Could you check a few things on this drawing? It's one solid part, dimensions in mm from its lowest x, y, z. A direction names the side the tool comes from. Give positions to 0.01 mm unless a question says otherwise; leave off trailing zeros. Order: outer loops, then holes, each group sorted by start corner. A loop starts at its lowest first (then second) coordinate and runs counter-clockwise, first axis right, second up.
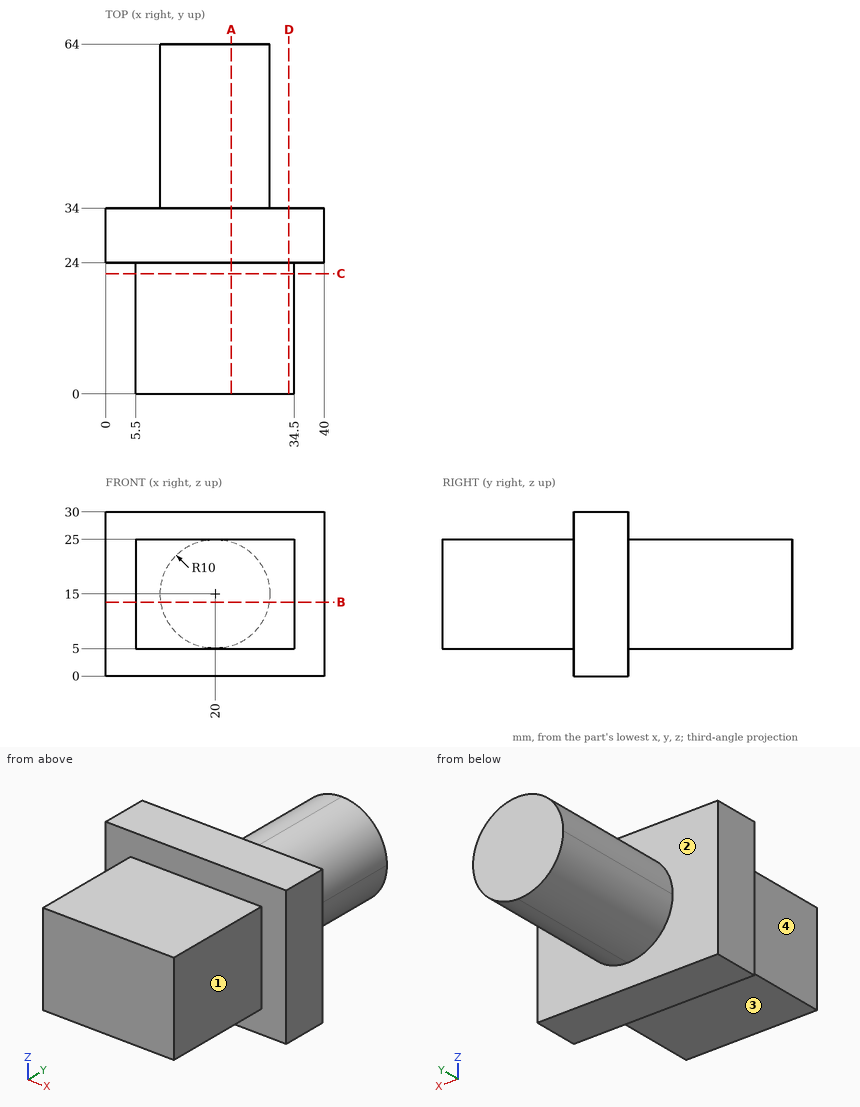
Q1. If we section it at D-D on x = 33.5: List the corners of the cut face in (y, z) for me.
Filled sheet:
outline: (0, 5) - (24, 5) - (24, 0) - (34, 0) - (34, 30) - (24, 30) - (24, 25) - (0, 25) - close
Q2. If we section it at C-C on y = 22: List the corners of the cut face in (x, z) for me.
Filled sheet:
outline: (5.5, 5) - (34.5, 5) - (34.5, 25) - (5.5, 25) - close
Q3. For the marked faces 1, 2, 3 and 4, which set-ups out of +Z, -Z, +X, -X, +Y, -Y let a thin tool reach every point of the face, with its end or its side?
Filled sheet:
face 1: +Z, -Z, +X, -Y
face 2: +Y
face 3: -Z, +X, -X, -Y
face 4: +Z, -Z, -X, -Y
Q4. If we section it at A-A on x = 23: List the corners of the cut face in (y, z) for me.
Filled sheet:
outline: (0, 5) - (24, 5) - (24, 0) - (34, 0) - (34, 5.46) - (64, 5.46) - (64, 24.54) - (34, 24.54) - (34, 30) - (24, 30) - (24, 25) - (0, 25) - close
Q5. I need wall thicknesses on L1, parallel to Z at x = 17, y = 13.5; L2, parallel to X at y = 11.5, z = 14.25; L3, parallel to Y at x = 15, z = 5.5. Which ranges of each line are inside material? Lowest first, please.
Filled sheet:
L1: z = 5 to 25
L2: x = 5.5 to 34.5
L3: y = 0 to 34
Q6. If we section it at B-B on z = 13.5: List the corners of the cut face in (x, y) for me.
Filled sheet:
outline: (0, 24) - (5.5, 24) - (5.5, 0) - (34.5, 0) - (34.5, 24) - (40, 24) - (40, 34) - (29.89, 34) - (29.89, 64) - (10.11, 64) - (10.11, 34) - (0, 34) - close
Q7. I'm going to push flat-ended pins straight in: P1, Ø7, axis at x = 24, y = 8, coming from the +Z side; P2, Ø4, axis at x = 30.5, y = 57.5, coming from the +Z side; P3, Ø5, axis at y = 51, z = 19.5, coming from the -X side; P4, Ø2, axis at x = 15.5, y = 28, coming from the -Z side. Where does each tip first touch, or does it pass through?
Filled sheet:
P1: stops at z = 25
P2: stops at z = 20.27
P3: stops at x = 10.2
P4: stops at z = 0
